from build123d import *

# Parameters (mm, degrees)
SKETCH1_W                = 44
SKETCH1_H                = 44
BOSS_EXTRUDE1_DEPTH      = 3
SKETCH2_R                = 3
BOSS_EXTRUDE2_DEPTH      = 7
BOSS_EXTRUDE2_TAPER      = 7
SKETCH4_R                = 2.5
CUT_EXTRUDE1_DEPTH       = 32.89043746
FILLET2_R                = 1
CIRPATTERN1_COUNT        = 4
FILLET2_OF_CIRPATTERN1_R = 1
FILLET3_R                = 1


with BuildPart() as part:
    # Sketch1 → Boss-Extrude1 (new body)
    with BuildSketch(Plane(origin=(0, 0, 0), x_dir=(1, 0, 0), z_dir=(0, 1, 0))):
        Rectangle(SKETCH1_W, SKETCH1_H)
    extrude(amount=BOSS_EXTRUDE1_DEPTH)

    # Sketch2 → Boss-Extrude2 (add)
    with BuildSketch(Plane(origin=(0, 3, 0), x_dir=(1, 0, 0), z_dir=(0, 1, 0))):
        with Locations((-17.7, 17.7)):
            Circle(SKETCH2_R)
    boss_extrude2 = extrude(amount=BOSS_EXTRUDE2_DEPTH, taper=BOSS_EXTRUDE2_TAPER)

    # Sketch3 → Cut-Revolve1 (revolve, cut)
    with BuildSketch(Plane(origin=(-17.7, 0, 0), x_dir=(0, 1, 0), z_dir=(-1, 0, 0)), mode=Mode.PRIVATE) as cut_revolve1_sk:
        Polygon((0, 17.7), (0, 20.5), (1.8, 20.182611435), (3.8, 20.182611435), (3.8, 19.4), (10, 19.4), (10, 17.7), align=None)
    cut_revolve1 = revolve(cut_revolve1_sk.sketch.rotate(Axis((-17.7, 10, -17.7), (0, -1, 0)), 180), axis=Axis((-17.7, 10, -17.7), (0, -1, 0)), mode=Mode.SUBTRACT)

    # Sketch4 → Cut-Extrude1 (cut, through all)
    with BuildSketch(Plane(origin=(0, 3, 0), x_dir=(1, 0, 0), z_dir=(0, 1, 0))):
        with Locations(Location((0, 0, 0), (0, 0, 270))):
            Circle(SKETCH4_R)
        Polygon((-14.871572875, 17.7), (-2, 17.7), (-2, 4.828427125), align=None)
        Polygon((-17.7, 2), (-4.828427125, 2), (-17.7, 14.871572875), align=None)
    cut_extrude1 = extrude(amount=-CUT_EXTRUDE1_DEPTH, mode=Mode.SUBTRACT)

    # Fillet2
    # the kernel refuses this fillet: 1 mm, written as the material it adds along each edge
    with BuildSketch(Plane(origin=(-2, 3, -4.828427125), x_dir=(0, 0, -1), z_dir=(0, -1, 0)), Plane(origin=(-14.871572875, 3, -17.7), x_dir=(0.7071067811865476, 0, 0.7071067811865476), z_dir=(0, -1, 0)), Plane(origin=(-17.7, 3, -14.871572875), x_dir=(0, 0, 1), z_dir=(0, -1, 0))) as fillet2_piece_1:
        with BuildLine():
            CenterArc((FILLET2_R * 2.41421356237, -FILLET2_R), FILLET2_R, 90, 135)
            Line((FILLET2_R * 1.70710678119, -FILLET2_R * 1.70710678119), (0, 0))
            Line((0, 0), (FILLET2_R * 2.41421356237, 0))
        make_face()
    extrude(amount=3)
    with BuildSketch(Plane(origin=(-2, 3, -17.7), x_dir=(0, 0, 1), z_dir=(0, -1, 0))) as fillet2_piece_2:
        with BuildLine():
            CenterArc((FILLET2_R, FILLET2_R), FILLET2_R, 180, 90)
            Line((0, FILLET2_R), (0, 0))
            Line((0, 0), (FILLET2_R, 0))
        make_face()
    extrude(amount=3)
    with BuildSketch(Plane(origin=(-17.7, 3, -2), x_dir=(1, 0, 0), z_dir=(0, -1, 0))) as fillet2_piece_3:
        with BuildLine():
            CenterArc((FILLET2_R, -FILLET2_R), FILLET2_R, 90, 90)
            Line((0, -FILLET2_R), (0, 0))
            Line((0, 0), (FILLET2_R, 0))
        make_face()
    extrude(amount=3)
    with BuildSketch(Plane(origin=(-4.828427125, 3, -2), x_dir=(-1, 0, 0), z_dir=(0, -1, 0))) as fillet2_piece_4:
        with BuildLine():
            CenterArc((FILLET2_R * 2.41421356237, FILLET2_R), FILLET2_R, 135, 135)
            Line((FILLET2_R * 1.70710678119, FILLET2_R * 1.70710678119), (0, 0))
            Line((0, 0), (FILLET2_R * 2.41421356237, 0))
        make_face()
    extrude(amount=3)

    # CirPattern1: Boss-Extrude2, Cut-Revolve1, Cut-Extrude1 ×4 about axis
    cirpattern1_axis = Axis((0, 0, 0), (0, 1, 0))
    add([boss_extrude2.rotate(cirpattern1_axis, i * 360 / CIRPATTERN1_COUNT) for i in range(1, CIRPATTERN1_COUNT)])
    add([cut_revolve1.rotate(cirpattern1_axis, i * 360 / CIRPATTERN1_COUNT) for i in range(1, CIRPATTERN1_COUNT)], mode=Mode.SUBTRACT)
    add([cut_extrude1.rotate(cirpattern1_axis, i * 360 / CIRPATTERN1_COUNT) for i in range(1, CIRPATTERN1_COUNT)], mode=Mode.SUBTRACT)

    # Fillet2 of CirPattern1
    # the kernel refuses this fillet: 1 mm, written as the material it adds along each edge
    with BuildSketch(Plane(origin=(-4.828427125, 3, 2), x_dir=(-1, 0, 0), z_dir=(0, -1, 0)), Plane(origin=(-2, 3, 4.828427125), x_dir=(-0.7071067811865477, 0, 0.7071067811865475), z_dir=(0, -1, 0)), Plane(origin=(2, 3, 4.828427125), x_dir=(0, 0, 1), z_dir=(0, -1, 0)), Plane(origin=(4.828427125, 3, 2), x_dir=(0.7071067811865475, 0, 0.7071067811865475), z_dir=(0, -1, 0)), Plane(origin=(4.828427125, 3, -2), x_dir=(1, 0, 0), z_dir=(0, -1, 0)), Plane(origin=(2, 3, -4.828427125), x_dir=(0.7071067811865476, 0, -0.7071067811865476), z_dir=(0, -1, 0))) as fillet2_of_cirpattern1_piece_1:
        with BuildLine():
            CenterArc((FILLET2_OF_CIRPATTERN1_R * 2.41421356237, -FILLET2_OF_CIRPATTERN1_R), FILLET2_OF_CIRPATTERN1_R, 90, 135)
            Line((FILLET2_OF_CIRPATTERN1_R * 1.70710678119, -FILLET2_OF_CIRPATTERN1_R * 1.70710678119), (0, 0))
            Line((0, 0), (FILLET2_OF_CIRPATTERN1_R * 2.41421356237, 0))
        make_face()
    extrude(amount=3)
    with BuildSketch(Plane(origin=(-17.7, 3, 14.871572875), x_dir=(0, 0, -1), z_dir=(0, -1, 0)), Plane(origin=(-14.871572875, 3, 17.7), x_dir=(0.7071067811865471, 0, -0.7071067811865479), z_dir=(0, -1, 0)), Plane(origin=(14.871572875, 3, 17.7), x_dir=(-1, 0, 0), z_dir=(0, -1, 0)), Plane(origin=(17.7, 3, 14.871572875), x_dir=(-0.7071067811865469, 0, -0.7071067811865483), z_dir=(0, -1, 0)), Plane(origin=(17.7, 3, -14.871572875), x_dir=(0, 0, 1), z_dir=(0, -1, 0)), Plane(origin=(14.871572875, 3, -17.7), x_dir=(-0.7071067811865487, 0, 0.7071067811865465), z_dir=(0, -1, 0))) as fillet2_of_cirpattern1_piece_2:
        with BuildLine():
            CenterArc((FILLET2_OF_CIRPATTERN1_R * 2.41421356237, FILLET2_OF_CIRPATTERN1_R), FILLET2_OF_CIRPATTERN1_R, 135, 135)
            Line((FILLET2_OF_CIRPATTERN1_R * 1.70710678119, FILLET2_OF_CIRPATTERN1_R * 1.70710678119), (0, 0))
            Line((0, 0), (FILLET2_OF_CIRPATTERN1_R * 2.41421356237, 0))
        make_face()
    extrude(amount=3)
    with BuildSketch(Plane(origin=(-17.7, 3, 2), x_dir=(1, 0, 0), z_dir=(0, -1, 0)), Plane(origin=(-2, 3, 17.7), x_dir=(-1, 0, 0), z_dir=(0, -1, 0)), Plane(origin=(2, 3, 17.7), x_dir=(0, 0, -1), z_dir=(0, -1, 0)), Plane(origin=(17.7, 3, 2), x_dir=(0, 0, 1), z_dir=(0, -1, 0)), Plane(origin=(17.7, 3, -2), x_dir=(-1, 0, 0), z_dir=(0, -1, 0)), Plane(origin=(2, 3, -17.7), x_dir=(1, 0, 0), z_dir=(0, -1, 0))) as fillet2_of_cirpattern1_piece_3:
        with BuildLine():
            CenterArc((FILLET2_OF_CIRPATTERN1_R, FILLET2_OF_CIRPATTERN1_R), FILLET2_OF_CIRPATTERN1_R, 180, 90)
            Line((0, FILLET2_OF_CIRPATTERN1_R), (0, 0))
            Line((0, 0), (FILLET2_OF_CIRPATTERN1_R, 0))
        make_face()
    extrude(amount=3)

    # Fillet3
    fillet3_edges = [part.edges().sort_by_distance(p)[0] for p in [
        (-17.7, 3, 20.7),
        (20.7, 3, 17.7),
        (17.7, 3, -20.7),
        (-20.7, 3, -17.7),
    ]]
    fillet(fillet3_edges, radius=FILLET3_R)


solid = part.part
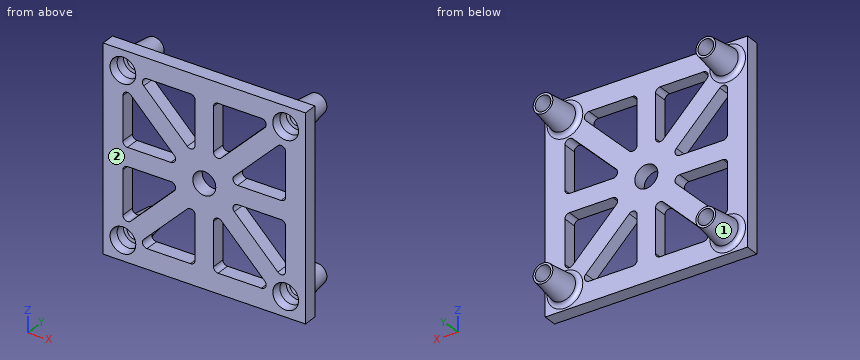
Geometry: final body of the model. Coordinates: model frame, mm. Face numbers are marked on the shaded views. Round coordinates to 2 decimals unless told otherwise and drop trailing zeros. Order: outer loops, then holes, each group sorted by start corner. A loop starts at its lowest first (then second) coordinate and runs counter-clockwise, first axis right, second up. Notation, with made-up numbers: (24.25, 69.5) -> (83.25, 69.5) arc R16 cw to (83.25, 74.5) -> close; hole circle Ø10 at (-12.5, 11). An arc over 180 degrees is marked (long way). Put each result on its own line as item: value. Start each with the question number.
Q1. Pull-direction query (Z, two-part tool) for the marked faces 1 and 2; classes: +Z half, -Z half, draft (parallel to the pull), parting line (faces both ways), or undercut.
Q2. Section D-D on x = 8. Return the cut outline in (y, z), and give its area (3 significant figures).
Q3. Line query: probe 1 along Z at (x, y) = (17.5, 8); probe 2 along X at (y, z) = (1.75, -3); probe 3 along X at (y, z) = (0.75, 17.5). Output: solid intervals per line, ascending.
Q4. Section A-A on x = 0. Return the cut outline in (y, z), and give its area (3 significant figures).
Q5. First-contact query: pin 1 (4 mm diameter, centred on x = 16.5, y = 8.5, fed in from +Z); pin 2 (3 mm diameter, centred on x = -10.5, z = -2, fed in from +Y). Flat tips, straight axial feed; report the tip coordinate or a pass-through.
Q6. Section B-B on z = 0. Return the cut outline in (x, y), and give its area (3 significant figures).
Q7. Section C-C on y = 6.25. Return the cut outline in (x, z).
Ans:
1. face 1: undercut
1. face 2: draft
2. outline: (0, -22) -> (3, -22) -> (3, -17.7) -> (0, -17.7) -> close; (0, -10.83) -> (3, -10.83) -> (3, -5.17) -> (0, -5.17) -> close; (0, -2) -> (3, -2) -> (3, 2) -> (0, 2) -> close; (0, 5.17) -> (3, 5.17) -> (3, 10.83) -> (0, 10.83) -> close; (0, 17.7) -> (3, 17.7) -> (3, 22) -> (0, 22) -> close
2. area: 71.7 mm2
3. probe 1: z = -20.08 to -19.39, -16.01 to -15.32, 15.32 to 16.01, 19.39 to 20.08
3. probe 2: x = -22 to -17.7, -6.24 to 6.24, 17.7 to 22
3. probe 3: x = -22 to -20.36, -15.04 to -13.06, -2.4 to 2.4, 13.06 to 15.04, 20.36 to 22
4. outline: (0, -22) -> (3, -22) -> (3, -2.5) -> (0, -2.5) -> close; (0, 2.5) -> (3, 2.5) -> (3, 22) -> (0, 22) -> close
4. area: 117 mm2
5. pin 1: stops at z = 20.23
5. pin 2: stops at y = 3
6. outline: (-22, 0) -> (-2.5, 0) -> (-2.5, 3) -> (-22, 3) -> close; (2.5, 0) -> (22, 0) -> (22, 3) -> (2.5, 3) -> close
6. area: 117 mm2
7. outline: circle Ø5.2 at (-17.7, -17.7); circle Ø5.2 at (-17.7, 17.7); circle Ø5.2 at (17.7, -17.7); circle Ø5.2 at (17.7, 17.7); hole circle Ø3.4 at (-17.7, -17.7); hole circle Ø3.4 at (-17.7, 17.7); hole circle Ø3.4 at (17.7, -17.7); hole circle Ø3.4 at (17.7, 17.7)
